Design review of the part shown in the three views and the two pictorial views. Dimensions are in mm from the part's minimum x, y and z. Give positions to 0.01 mm unless a question says otherwise; leave off trailing zeros. Order: outer loops, then holes, each group sorted by start corner. A loop starts at its lowest first (then second) coordinate and runs counter-clockwise, first axis right, second up.
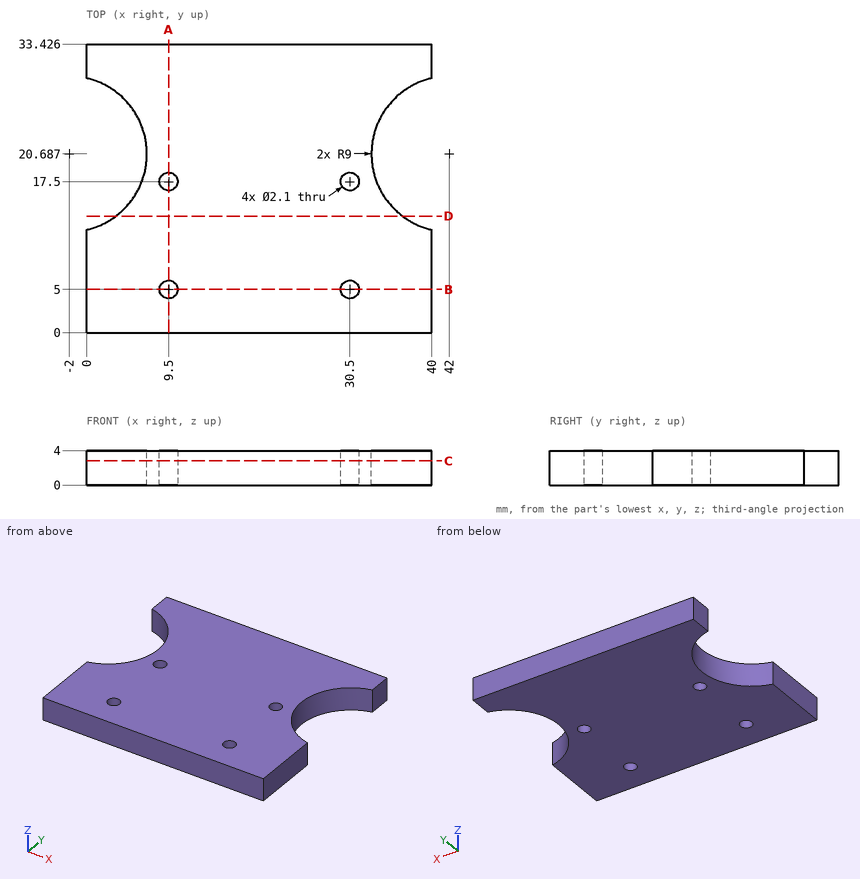
1) We need section D-D on y = 13.5. Give the boundary of the cut face in (x, z).
Answer sheet:
outline: (3.42, 0) - (36.58, 0) - (36.58, 4) - (3.42, 4) - close
2) To check wall thickness, follow line 1 (Y direction, x = 9.5, z = 1.35); line 2 (X direction, y = 18, z = 3.25) (1 decimal); line 3 (X direction, y = 17, z = 2.9) (1 decimal). State the ranges of each line that lie inside material, in increasing order.
Answer sheet:
line 1: y = 0 to 3.95, 6.05 to 16.45, 18.55 to 33.43
line 2: x = 6.6 to 8.6, 10.4 to 29.6, 31.4 to 33.4
line 3: x = 6.2 to 8.6, 10.4 to 29.6, 31.4 to 33.8
3) We need section A-A on x = 9.5. Give the boundary of the cut face in (y, z).
Answer sheet:
outline: (0, 0) - (3.95, 0) - (3.95, 4) - (0, 4) - close; (6.05, 0) - (16.45, 0) - (16.45, 4) - (6.05, 4) - close; (18.55, 0) - (33.43, 0) - (33.43, 4) - (18.55, 4) - close
4) We need section B-B on y = 5. Give the boundary of the cut face in (x, z), then the cut area to 3 significant figures.
Answer sheet:
outline: (0, 0) - (8.45, 0) - (8.45, 4) - (0, 4) - close; (10.55, 0) - (29.45, 0) - (29.45, 4) - (10.55, 4) - close; (31.55, 0) - (40, 0) - (40, 4) - (31.55, 4) - close
area: 143 mm2
5) Clearance check with a flat-ended pin moving along its axis: pin 1 (1.3 mm diameter, centred on x = 30.5, y = 17.5, fed in from +Z). State where the tip first meets the part, or that it passes through.
Answer sheet:
pin 1: passes through
6) We need section C-C on z = 2.8. Give the boundary of the cut face in (x, y), then the cut area to 3 significant figures.
Answer sheet:
outline: (0, 0) - (40, 0) - (40, 11.91) arc R9 cw to (40, 29.46) - (40, 33.43) - (0, 33.43) - (0, 29.46) arc R9 cw to (0, 11.91) - close; hole circle Ø2.1 at (9.5, 5); hole circle Ø2.1 at (9.5, 17.5); hole circle Ø2.1 at (30.5, 5); hole circle Ø2.1 at (30.5, 17.5)
area: 1,140 mm2
